Model file for the job. Use its own axes, mm. Face numbers are marked on the shaded views. Coordinates: 2 decimals unless noted, no trailing zeros. Order: outer loops, then holes, each group sorted by start corner. A loop starts at its lowest first (then second) coordinate and runs counter-clockwise, first axis right, second up.
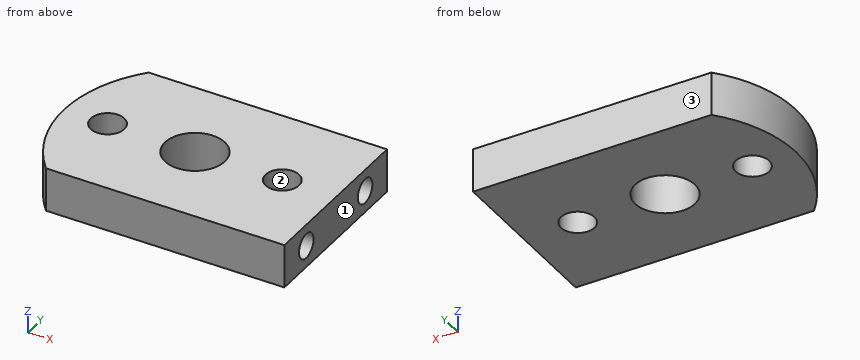
from build123d import *

# Parameters (mm, degrees)
SKETCH1_W                     = 44.45
SKETCH1_H                     = 23.0124
BOSS_EXTRUDE1_DEPTH           = 4.7625
F_1_4_CLEARANCE_HOLE1_D       = 6.5278
F_6_CLEARANCE_HOLE1_D         = 3.6576
CUT_EXTRUDE1_DEPTH            = 51.279761933
TAP_DRILL_FOR_6_32_TAP1_D     = 2.7051
TAP_DRILL_FOR_6_32_TAP1_DEPTH = 12.7
TAP_DRILL_FOR_6_32_TAP1_TIP   = 0.81269403


with BuildPart() as part:
    # Sketch1 → Boss-Extrude1 (new body)
    with BuildSketch(Plane.XY):
        with Locations((22.225, 11.5062)):
            Rectangle(SKETCH1_W, SKETCH1_H)
    extrude(amount=BOSS_EXTRUDE1_DEPTH)

    # 1/4 Clearance Hole1 (through all)
    with Locations(Plane.XY.offset(4.7625)):
        with Locations((29.1015, 10.3124)):
            Hole(F_1_4_CLEARANCE_HOLE1_D / 2)

    # #6 Clearance Hole1 (through all)
    with Locations(Plane.XY.offset(4.7625)):
        with Locations((19.5765, 10.3124), (38.6265, 10.3124)):
            Hole(F_6_CLEARANCE_HOLE1_D / 2)

    # Sketch7 → Cut-Extrude1 (cut, through all)
    with BuildSketch(Plane.XY.offset(4.7625)):
        with BuildLine():
            Line((18.452226257, 0.7874), (44.45, 0.7874))
            Line((44.45, 0.7874), (44.45, 0))
            Line((44.45, 0), (0, 0))
            Line((0, 0), (0, 23.0124))
            Line((0, 23.0124), (44.45, 23.0124))
            Line((44.45, 23.0124), (44.45, 19.8374))
            Line((44.45, 19.8374), (18.452226257, 19.8374))
            ThreePointArc((18.452226257, 19.8374), (14.814, 10.3124), (18.452226257, 0.7874))
        make_face()
    extrude(amount=-CUT_EXTRUDE1_DEPTH, mode=Mode.SUBTRACT)

    # Tap Drill for #6-32 Tap1
    with Locations(Plane(origin=(44.45, 0, 0), x_dir=(0, 0, -1), z_dir=(1, 0, 0))):
        with Locations((-2.38125, 4.8514), (-2.38125, 15.7734)):
            Hole(TAP_DRILL_FOR_6_32_TAP1_D / 2, depth=TAP_DRILL_FOR_6_32_TAP1_DEPTH)
            with Locations((0, 0, -(TAP_DRILL_FOR_6_32_TAP1_DEPTH + TAP_DRILL_FOR_6_32_TAP1_TIP / 2))):  # 118° drill point
                Cone(0, TAP_DRILL_FOR_6_32_TAP1_D / 2, TAP_DRILL_FOR_6_32_TAP1_TIP, mode=Mode.SUBTRACT)


solid = part.part
Q1. Drop a flat-ended pin along its axis: P1, Ø2, axis at y = 15.77, z = 2.38, coming from the +X side. Give the stop position or say it passes through.
Established:
P1: stops at x = 31.54
Q2. Cut at C-C, the plane z = 0.7. Count the separate pieces of the cut face and the enclosed holes in it, plus the area to 3 significant figures.
Established:
separate pieces: 1
enclosed holes: 3
area: 488 mm2
Q3. Cut at D-D, the plane x = 41. List the corners of the cut face in (y, z).
Established:
outline: (0.79, 0) - (19.84, 0) - (19.84, 4.76) - (0.79, 4.76) - close; hole circle Ø2.71 at (4.85, 2.38); hole circle Ø2.71 at (15.77, 2.38)
Q4. Cut at B-B, the plane x = 20.5. List the corners of the cut face in (y, z).
Established:
outline: (0.79, 0) - (8.73, 0) - (8.73, 4.76) - (0.79, 4.76) - close; (11.89, 0) - (19.84, 0) - (19.84, 4.76) - (11.89, 4.76) - close
Q5. Cut at A-A, the plane x = 37.75. List the corners of the cut face in (y, z).
Established:
outline: (0.79, 0) - (8.71, 0) - (8.71, 4.76) - (0.79, 4.76) - close; (11.92, 0) - (19.84, 0) - (19.84, 4.76) - (11.92, 4.76) - close; hole circle Ø2.71 at (4.85, 2.38); hole circle Ø2.71 at (15.77, 2.38)
Q6. Probe line 1 (X direction, y = 10.25, z = 0.7); line 2 (X direction, y = 7.5, z = 3.2); line 3 (X direction, y = 12.5, z = 4.1). List the from-to ranges inside material, lowest first.
Established:
line 1: x = 14.81 to 17.75, 21.4 to 25.84, 32.36 to 36.8, 40.45 to 44.45
line 2: x = 15.09 to 27.45, 30.76 to 44.45
line 3: x = 14.98 to 26.68, 31.52 to 44.45
Q7. Mould opens along X. For the marked faces 1, 2 and 3 say: pulls with the +X half, pulls with the -X half, needs draft (parallel to the pull), parting line crosses it, or undercut.
Established:
face 1: pulls with the +X half
face 2: undercut
face 3: needs draft
